Print and shaded views of the part. All mm, measured from the part's lowest x, y and z. A direction names the side the tool comes from. Coordinates: 2 decimals unless noted, no trailing zeros. Loops run counter-clockwise (first coordinate to the right, second up) from the corner with the lowest first, then second, coordinate; pieces in that order, holes last. Notation, with made-up numbers: M -40,3 L 11,3 A32 ccw 11,36 Z; hole C 9.25,-27.75 d6. An arc over 180 degrees is marked long. Answer as a JSON object with one key per item and string values. Group by question number.
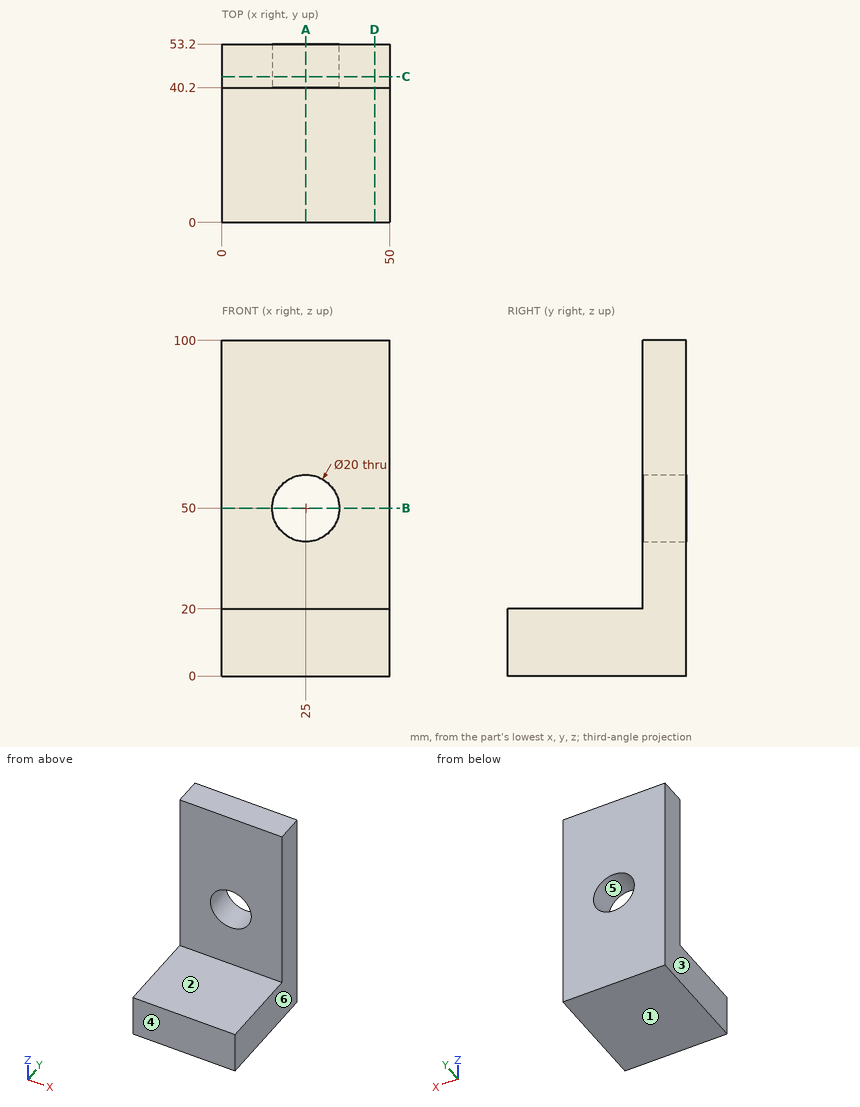
Item 1: Drill centre lines: L1, parallel to Z at x = 25, y = 50; L2, parallel to Z at x = 29, y = 3; L3, parallel to Y at x = 34, z = 62. Where is each one in solid material? Low to high. Write a range as from..to.
Item 2: Pull direction X, two halves, no side cores. Call the marked faces 3, 4, 5 and 6: released by +X, released by -X, zero draft, split by the parting line, or undercut.
Item 3: Slice it at C-C, the plane y = 43.5. Write the cut outline in (x, z).
Item 4: Pin check, flat tips, straight feed: pin 1 (4 mm diameter, centred on x = 43.5, z = 58.5, fed in from -Y); pin 2 (8 mm diameter, centred on x = 14, z = 23, fed in from -Y). Stop position of each tip, or through.
Item 5: Slice it at B-B, the plane z = 50. Write the cut outline in (x, y), then the cut area to 3 significant figures.
Item 6: Tool access for the marked faces 1 and 2: list every direction of +Z, -Z, +X, -X, +Y, -Y with a clear straight run to the whole face (end or side of a thin tool).
Item 7: Slice it at D-D, the plane x = 45.5. Write the cut outline in (y, z), then the cut area to 3 significant figures.
Item 8: Slice it at A-A, the plane x = 25. Write the cut outline in (y, z).
Computed:
{
 "1": {"L1": "0..40, 60..100", "L2": "0..20", "L3": "40.2..53.2"},
 "2": {"face 3": "released by -X", "face 4": "zero draft", "face 5": "undercut", "face 6": "released by +X"},
 "3": {"outline": "M 0,0 L 50,0 L 50,100 L 0,100 Z; hole C 25,50 d20"},
 "4": {"pin 1": "y = 40.2", "pin 2": "y = 0"},
 "5": {"outline": "M 0,40.2 L 15,40.2 L 15,53.2 L 0,53.2 Z; M 35,40.2 L 50,40.2 L 50,53.2 L 35,53.2 Z", "area": "390 mm2"},
 "6": {"face 1": "-Z, +X, -X, +Y, -Y", "face 2": "+Z, +X, -X, -Y"},
 "7": {"outline": "M 0,0 L 53.2,0 L 53.2,100 L 40.2,100 L 40.2,20 L 0,20 Z", "area": "2,100 mm2"},
 "8": {"outline": "M 0,0 L 53.2,0 L 53.2,40 L 40.2,40 L 40.2,20 L 0,20 Z; M 40.2,60 L 53.2,60 L 53.2,100 L 40.2,100 Z"}
}
